from build123d import *

# Parameters (mm, degrees)
SKETCH1_W               = 38
SKETCH1_H               = 110
BOSS_EXTRUDE1_DEPTH     = 2.5
CUT_EXTRUDE1_DEPTH      = 59.243025334
CUT_EXTRUDE1_DEPTH_BACK = 59.243025334
SKETCH2_R               = 2.25


with BuildPart() as part:
    # Sketch1 → Boss-Extrude1 (new body)
    with BuildSketch(Plane.XY):
        Rectangle(SKETCH1_W, SKETCH1_H)
    extrude(amount=BOSS_EXTRUDE1_DEPTH)

    # Sketch2 → Cut-Extrude1 (cut, two sides: drawn at the far end of the back side and taken through both)
    with BuildSketch(Plane.XY.offset(2.5).offset(-CUT_EXTRUDE1_DEPTH_BACK)):
        with Locations((0, 35)):
            Circle(SKETCH2_R)
        with Locations((0, -35)):
            Circle(SKETCH2_R)
    extrude(amount=CUT_EXTRUDE1_DEPTH + CUT_EXTRUDE1_DEPTH_BACK, mode=Mode.SUBTRACT)


solid = part.part
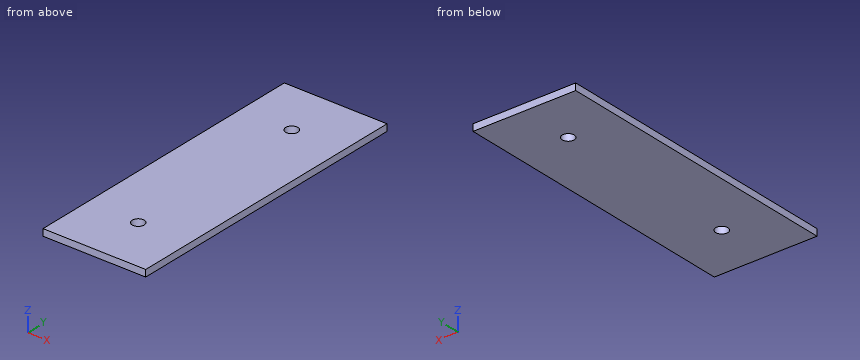
Geometry: final body of the model. Coordinates: model frame, mm. Give positions to 0.01 mm unless a question says otherwise; leave off trailing zeros. Loops run counter-clockwise (first coordinate to the right, second up) from the corner with the lowest first, then second, coordinate; pieces in that order, holes last. Notation, with made-up numbers: (62, 10) - (69, 10) arc R31 cw to (69, 37) - close; hole circle Ø3 at (-19.75, -26.5). An arc over 180 degrees is marked (long way). Answer as CSV lines item,"result". Start each with the question number.
1. Ray query, L1, parallel to Y at x = 0, z = 0.75; L2, parallel to X at y = 35, z = 0.65; L3, parallel to Y at x = 2, z = 0.2. Return the intervals inside material, ascending.
2. Section B-B, the plane x = 0. Return loops of the section in (y, z).
3. Section A-A, the plane y = -35. Return loops of the section in (x, z).
Answers:
1,L1,"y = -55 to -37.25, -32.75 to 32.75, 37.25 to 55"
1,L2,"x = -19 to -2.25, 2.25 to 19"
1,L3,"y = -55 to -36.03, -33.97 to 33.97, 36.03 to 55"
2,outline,"(-55, 0) - (-37.25, 0) - (-37.25, 2.5) - (-55, 2.5) - close; (-32.75, 0) - (32.75, 0) - (32.75, 2.5) - (-32.75, 2.5) - close; (37.25, 0) - (55, 0) - (55, 2.5) - (37.25, 2.5) - close"
3,outline,"(-19, 0) - (-2.25, 0) - (-2.25, 2.5) - (-19, 2.5) - close; (2.25, 0) - (19, 0) - (19, 2.5) - (2.25, 2.5) - close"
